Geometry check sheet. Reference: the model listing, model coordinates, mm. A direction names the side the tool comes from. Round coordinates to 2 decimals unless told otherwise and drop trailing zeros. Order: outer loops, then holes, each group sorted by start corner. A loop starts at its lowest first (then second) coordinate and runs counter-clockwise, first axis right, second up. Notation, with made-up numbers: (-31, 79) -> (-5, 79) arc R9 ccw to (-5, 96) -> close; hole circle Ø6 at (24.5, 22). An arc over 180 degrees is marked (long way). Use a Markdown table: item, result. Add a question column.
Item 1: Mould release check, pull along X, two halves, no side actions. Record for faces 1 (the cylindrical face through (180.14, 4.1, 27.99)), 2 (the cylindrical face through (4.35, -1.23, 16.07)), 3 (the flat face through (89, 0, 35)): pulls with the +X half, pulls with the -X half, needs draft (parallel to the pull), parting line crosses it, or undercut.
Item 2: Set-up check for faces 4 (the flat face through (181, -1, 21)), 5 (the flat face through (89, 3, 29)), 6 (the flat face through (89, 0, 8)): record each of +Z, -Z, +X, -X, +Y, -Y from which the full face is reachable in a straight line by a thin tool's end or side.
Item 3: Material ranges on probe 1 along Z at (x, y) = (5, -1.55); probe 2 along Z at (x, y) = (175, -1.65); probe 3 along Y at (x, z) = (60.5, 10), recorded low to high. Write a range as [from, to].
Item 4: Gauge pin test, flat ends, axial feed: pin 1 Ø1.2 at (x, y) = (164.5, -1) entering from -Z; pin 2 Ø8 at (x, z) = (62, 11.5) entering from +Y; pin 3 Ø5 at (x, z) = (175, 13) entering from +Y. Record the tip position at first contact, or that the pin passes through.
Item 5: Sectioned sample at D-D, the plane x = 129.5. Record the cut outline in (y, z).
Item 6: Sectioned sample at B-B, the plane z = 19. Record the cut outline in (x, y), and give its area (3 significant figures).
Item 7: Sectioned sample at C-C, the plane x = 69. Record the cut outline in (y, z).
Item 8: Sectioned sample at A-A, the plane x = 175. Record the cut outline in (y, z), and give its area (3 significant figures).
from build123d import *

# Parameters (mm, degrees)
SKETCH_W     = 181
SKETCH_H     = 42
SKETCH_R     = 3
SKETCH_W_2   = 9
SKETCH_H_2   = 11
SKETCH_W_3   = 12.5
SKETCH_H_3   = 1.5
SKETCH_W_4   = 16.5
SKETCH_H_4   = 14
PAD_DEPTH    = 2.5
PAD001_DEPTH = 2
PAD002_DEPTH = 2


with BuildPart() as part:
    # Sketch → Pad (new body)
    with BuildSketch(Plane.XZ):
        with Locations((90.5, 21)):
            Rectangle(SKETCH_W, SKETCH_H)
        with Locations((175, 13)):
            Circle(SKETCH_R, mode=Mode.SUBTRACT)
        with Locations((5, 19)):
            Circle(SKETCH_R, mode=Mode.SUBTRACT)
        with Locations((162.5, 15.75)):
            Rectangle(SKETCH_W_2, SKETCH_H_2, mode=Mode.SUBTRACT)
        with BuildLine():
            Line((96, 26.75), (107.5, 26.75))
            ThreePointArc((109.5, 24.75), (108.914214, 26.164214), (107.5, 26.75))
            Line((109.5, 24.75), (109.5, 12.25))
            ThreePointArc((107.5, 10.25), (108.914214, 10.835786), (109.5, 12.25))
            Line((107.5, 10.25), (96, 10.25))
            ThreePointArc((94, 12.25), (94.585786, 10.835786), (96, 10.25))
            Line((94, 12.25), (94, 24.75))
            ThreePointArc((96, 26.75), (94.585786, 26.164214), (94, 24.75))
        make_face(mode=Mode.SUBTRACT)
        with Locations((130.25, 11)):
            Rectangle(SKETCH_W_3, SKETCH_H_3, mode=Mode.SUBTRACT)
        with BuildLine():
            Line((112.5, 13.25), (121, 13.25))
            Line((121, 13.25), (121, 12.25))
            ThreePointArc((119, 10.25), (120.414214, 10.835786), (121, 12.25))
            Line((119, 10.25), (114.5, 10.25))
            ThreePointArc((112.5, 12.25), (113.085786, 10.835786), (114.5, 10.25))
            Line((112.5, 12.25), (112.5, 13.25))
        make_face(mode=Mode.SUBTRACT)
        with Locations((82.75, 17.25)):
            Rectangle(SKETCH_W_4, SKETCH_H_4, mode=Mode.SUBTRACT)
        with BuildLine():
            Line((49, 17), (64, 17))
            Line((64, 17), (64, 13))
            ThreePointArc((61.5, 10.5), (63.267767, 11.232233), (64, 13))
            Line((61.5, 10.5), (51.5, 10.5))
            ThreePointArc((49, 13), (49.732233, 11.232233), (51.5, 10.5))
            Line((49, 13), (49, 17))
        make_face(mode=Mode.SUBTRACT)
        with BuildLine():
            Line((24, 17), (39, 17))
            Line((39, 17), (39, 13))
            ThreePointArc((36.5, 10.5), (38.267767, 11.232233), (39, 13))
            Line((36.5, 10.5), (26.5, 10.5))
            ThreePointArc((24, 13), (24.732233, 11.232233), (26.5, 10.5))
            Line((24, 13), (24, 17))
        make_face(mode=Mode.SUBTRACT)
    extrude(amount=PAD_DEPTH)

    # Sketch001 (on Part) → Pad001 (join)
    with BuildSketch(Plane.XY.offset(27)):
        with BuildLine():
            Line((0, 0), (181, 0))
            Line((181, 0), (181, 2))
            ThreePointArc((181, 2), (180.12132, 4.12132), (178, 5))
            Line((178, 5), (3, 5))
            ThreePointArc((3, 5), (0.87868, 4.12132), (0, 2))
            Line((0, 2), (0, 0))
        make_face()
    extrude(amount=PAD001_DEPTH)

    # Sketch002 → Pad002 (join)
    with BuildSketch(Plane.XY.offset(40)):
        with BuildLine():
            Line((0, 0), (181, 0))
            Line((181, 0), (181, 2))
            ThreePointArc((181, 2), (180.12132, 4.12132), (178, 5))
            Line((178, 5), (3, 5))
            ThreePointArc((3, 5), (0.87868, 4.12132), (0, 2))
            Line((0, 2), (0, 0))
        make_face()
    extrude(amount=PAD002_DEPTH)


solid = part.part
Found:
| question | item | result |
|---|---|---|
| 1 | face 1 | pulls with the +X half |
| 1 | face 2 | undercut |
| 1 | face 3 | needs draft |
| 2 | face 4 | +Z, -Z, +X, +Y, -Y |
| 2 | face 5 | +X, -X, +Y |
| 2 | face 6 | -Z, +X, -X, +Y |
| 3 | probe 1 | z = [0, 16], [22, 42] |
| 3 | probe 2 | z = [0, 10], [16, 42] |
| 3 | probe 3 | y = [-2.5, 0] |
| 4 | pin 1 | stops at z = 0 |
| 4 | pin 2 | stops at y = 0 |
| 4 | pin 3 | passes through |
| 5 | outline | (-2.5, 0) -> (0, 0) -> (0, 10.25) -> (-2.5, 10.25) -> close; (-2.5, 11.75) -> (0, 11.75) -> (0, 27) -> (5, 27) -> (5, 29) -> (0, 29) -> (0, 40) -> (5, 40) -> (5, 42) -> (-2.5, 42) -> close |
| 6 | outline | (0, -2.5) -> (2, -2.5) -> (2, 0) -> (0, 0) -> close; (8, -2.5) -> (74.5, -2.5) -> (74.5, 0) -> (8, 0) -> close; (91, -2.5) -> (94, -2.5) -> (94, 0) -> (91, 0) -> close; (109.5, -2.5) -> (158, -2.5) -> (158, 0) -> (109.5, 0) -> close; (167, -2.5) -> (181, -2.5) -> (181, 0) -> (167, 0) -> close |
| 6 | area | 335 mm2 |
| 7 | outline | (-2.5, 0) -> (0, 0) -> (0, 27) -> (5, 27) -> (5, 29) -> (0, 29) -> (0, 40) -> (5, 40) -> (5, 42) -> (-2.5, 42) -> close |
| 8 | outline | (-2.5, 0) -> (0, 0) -> (0, 10) -> (-2.5, 10) -> close; (-2.5, 16) -> (0, 16) -> (0, 27) -> (5, 27) -> (5, 29) -> (0, 29) -> (0, 40) -> (5, 40) -> (5, 42) -> (-2.5, 42) -> close |
| 8 | area | 110 mm2 |
